```python
from build123d import *

# Parameters (mm, degrees)
CORTE_EXTRUS_O_FINA1_DEPTH = 9


with BuildPart() as part:
    # Esboço1 → Revolução1 (revolve)
    with BuildSketch(Plane.XY):
        Polygon((0, 0), (12.5, 0), (12.5, 40), (5.5, 40), (5.5, 42), (2, 42), (2, 52), (0, 52), align=None)
    revolve(axis=Axis((0, 52, 0), (0, -1, 0)))

    # Esboço2 → Corte-Extrusão-Fina1 (cut)
    with BuildSketch(Plane(origin=(0, 52, 0), x_dir=(1, 0, 0), z_dir=(0, 1, 0))):
        with BuildLine():
            Line((-4.795831523, 11), (4.795831523, 11))
            ThreePointArc((4.795831523, 11), (0, -12), (-4.795831523, 11))
        make_face()
        with BuildLine():
            Line((-1.732050808, 1), (1.732050808, 1))
            ThreePointArc((1.732050808, 1), (0, -2), (-1.732050808, 1))
        make_face(mode=Mode.SUBTRACT)
    extrude(amount=-CORTE_EXTRUS_O_FINA1_DEPTH, mode=Mode.SUBTRACT)


solid = part.part
```
Read the model definition and answer for the solid it produces. Units are mm, in the model's axes. A direction names the side the tool comes from. Give positions to 0.01 mm unless a question says otherwise; leave off trailing zeros. Order: outer loops, then holes, each group sorted by start corner. A loop starts at its lowest first (then second) coordinate and runs counter-clockwise, first axis right, second up.
(1) Straight lines are drawn through the part: L1, parallel to Y at x = -1, z = -3; L2, parallel to Y at x = 9.75, z = -4.5; L3, parallel to X at y = 28.5, z = -0.5. For each, find the intervals that lie inside material, in ascending order.
(2) Given pin 1 (2 mm diameter, centred on x = -8.5, z = 0, fed in from +Y); pin 2 (2 mm diameter, centred on y = 22, z = -6.5, fed in from -X) (3 decimals); pin 3 (5 mm diameter, centred on x = -4.5, z = -6, fed in from +Y), each flat-ended and moving along its own axis, determine where each tip first touches the part or whether it passes through.
(3) Find section B-B (z = 0). Give the vertices of the cut face in (x, y), plus the area to 3 significant figures.
(4) Find section C-C (y = 48.5). Give the vertices of the cut face in (x, z), plus the area to 3 significant figures.
(5) For faces 1 (the flat face through (0, 0, 0)), 2 (the cylindrical face through (0, 47, 2)), 3 (the flat face through (0, 48, -1)), determine the directions among +Z, -Z, +X, -X, +Y, -Y from which every point of the face is accessible in a straight line to the end or side of a thin tool.
(6) Find section A-A (x = 0). Give the vertices of the cut face in (y, z), plus the area to 3 significant figures.
(7) Find section D-D (x = 4). Give the vertices of the cut face in (y, z).
Result sheet:
1. L1: y = 0 to 42
1. L2: y = 0 to 40
1. L3: x = -12.49 to 12.49
2. pin 1: stops at y = 40
2. pin 2: stops at x = -11.225
2. pin 3: stops at y = 42
3. outline: (-12.5, 0) - (12.5, 0) - (12.5, 40) - (5.5, 40) - (5.5, 42) - (2, 42) - (2, 52) - (-2, 52) - (-2, 42) - (-5.5, 42) - (-5.5, 40) - (-12.5, 40) - close
3. area: 1,060 mm2
4. outline: (-1.73, -1) - (1.73, -1) arc R2 ccw (long way) to start
4. area: 10.1 mm2
5. face 1: +Z, -Z, +X, -X, -Y
5. face 2: +Y
5. face 3: -Z, +X, -X, +Y
6. outline: (0, -12.5) - (40, -12.5) - (40, -5.5) - (42, -5.5) - (42, -2) - (43, -2) - (43, -1) - (52, -1) - (52, 2) - (42, 2) - (42, 5.5) - (40, 5.5) - (40, 12.5) - (0, 12.5) - close
6. area: 1,050 mm2
7. outline: (0, -11.84) - (40, -11.84) - (40, -3.77) - (42, -3.77) - (42, 3.77) - (40, 3.77) - (40, 11.84) - (0, 11.84) - close
